Check sheet for the modelled part. Datum: model origin and axes. Units: mm. A direction names the side the tool comes from. Give positions to 0.01 mm unless a question says otherwise; leave off trailing zeros. Loops run counter-clockwise (first coordinate to the right, second up) from the corner with the lowest first, then second, coordinate; pieces in that order, holes last.
```python
from build123d import *

# Parameters (mm, degrees)
SKETCH_10_R         = 1.65
EXTRUDE_1_DEPTH     = 3
EXTRUDE_START       = 3
EXTRUDE_2_DEPTH     = 7
EXTRUDE_3_DEPTH     = 13
CHAMFER_1_SIZE      = 7
EXTRUDE_5_DEPTH     = 10
EXTRUDE_START_2     = -1.1
SKETCH_16_R         = 1.65
EXTRUDE_6_DEPTH     = 4.1
EXTRUDE_7_DEPTH     = 16
SKETCH_18_W         = 21
SKETCH_18_H         = 15.2
CUT_EXTRUDE_1_DEPTH = 14.1
FILLET_1_R          = 1


with BuildPart() as part:
    # 草图10 → 凸台-拉伸1 (new body)
    with BuildSketch(Plane.XY):
        Polygon((-78.55, -32.8), (-46.235028843, -32.8), (38.364971157, 51.8), (78.55, 51.8), (78.55, 32.8), (46.235028843, 32.8), (-38.364971157, -51.8), (-78.55, -51.8), align=None)
        with Locations((-68.55, -42.3)):
            Circle(SKETCH_10_R, mode=Mode.SUBTRACT)
        with Locations((68.55, 42.3)):
            Circle(SKETCH_10_R, mode=Mode.SUBTRACT)
    extrude(amount=EXTRUDE_1_DEPTH)

    # 草图11 → 凸台-拉伸2 (add)
    with BuildSketch(Plane.XY.offset(EXTRUDE_START)):
        Polygon((-59.55, -32.8), (-59.55, -51.8), (-38.364971157, -51.8), (46.235028843, 32.8), (57.55, 32.8), (57.55, 51.8), (38.364971157, 51.8), (-46.235028843, -32.8), align=None)
    extrude(amount=EXTRUDE_2_DEPTH)

    # 草图12 → 凸台-拉伸3 (add)
    with BuildSketch(Plane.XY.offset(EXTRUDE_START)):
        Polygon((-78.55, -32.8), (-46.235028843, -32.8), (38.364971157, 51.8), (78.55, 51.8), (78.55, 48.8), (39.607611845, 48.8), (-44.992388155, -35.8), (-78.55, -35.8), align=None)
        Polygon((-78.55, -48.8), (-78.55, -51.8), (-38.364971157, -51.8), (46.235028843, 32.8), (78.55, 32.8), (78.55, 35.8), (44.992388155, 35.8), (-39.607611845, -48.8), align=None)
    extrude(amount=EXTRUDE_3_DEPTH)

    # 倒角1
    chamfer_1_edges = [part.edges().sort_by_distance(p)[0] for p in [
        (57.55, 42.3, 10),
        (-59.55, -42.3, 10),
    ]]
    chamfer(chamfer_1_edges, length=CHAMFER_1_SIZE - 0.0001)  # a hair under: the kernel refuses the full size

    # 草图15 → 凸台-拉伸5 (add)
    with BuildSketch(Plane.XY.offset(3)):
        Polygon((-55.55, -35.8), (-55.55, -39.8), (-43.335533906, -39.8), (41.264466094, 44.8), (53.55, 44.8), (53.55, 48.8), (39.607611845, 48.8), (-44.992388155, -35.8), align=None)
        Polygon((-55.55, -44.8), (-55.55, -48.8), (-39.607611845, -48.8), (44.992388155, 35.8), (53.55, 35.8), (53.55, 39.8), (43.335533906, 39.8), (-41.264466094, -44.8), align=None)
    extrude(amount=EXTRUDE_5_DEPTH)

    # 草图16 → 凸台-拉伸6 (add)
    with BuildSketch(Plane.XY.offset(EXTRUDE_START_2)):
        Polygon((-78.55, -32.8), (-78.55, -51.8), (-38.364971157, -51.8), (45.135028843, 31.7), (78.55, 31.7), (78.55, 52.9), (39.464971157, 52.9), (-46.235028843, -32.8), align=None)
        with Locations((-68.55, -42.3)):
            Circle(SKETCH_16_R, mode=Mode.SUBTRACT)
        with Locations((68.55, 42.3)):
            Circle(SKETCH_16_R, mode=Mode.SUBTRACT)
    extrude(amount=EXTRUDE_6_DEPTH)

    # 草图17 → 凸台-拉伸7 (add)
    with BuildSketch(Plane.XY):
        Polygon((78.55, 52.9), (78.55, 48.8), (39.607611845, 48.8), (37.486291501, 50.921320344), (39.464971157, 52.9), align=None)
        Polygon((78.55, 31.7), (45.135028843, 31.7), (43.013708499, 33.821320344), (44.992388155, 35.8), (78.55, 35.8), align=None)
    extrude(amount=EXTRUDE_7_DEPTH)

    # 草图18 → 切除-拉伸1 (cut)
    with BuildSketch(Plane.XY.offset(16)):
        with Locations((68.05, 42.3)):
            Rectangle(SKETCH_18_W, SKETCH_18_H)
    extrude(amount=-CUT_EXTRUDE_1_DEPTH, mode=Mode.SUBTRACT)


with BuildPart() as cut_extrude_1_kept_piece:
    # of the separate pieces the step leaves, the one the design keeps (cut_extrude_1_pieces_kept)
    add(part.part.solids().sort_by_distance((-59.55, -48.8, 3.0001))[0])

    # 圆角1
    fillet_1_edges = [cut_extrude_1_kept_piece.edges().sort_by_distance(p)[0] for p in [
        (-46.235028843, -32.8, 7.45),
        (-38.364971157, -51.8, 7.45),
        (-43.335533906, -39.8, 11.5),
        (41.264466094, 44.8, 11.5),
        (-41.264466094, -44.8, 11.5),
        (43.335533906, 39.8, 11.5),
        (45.135028843, 31.7, 7.45),
        (39.464971157, 52.9, 7.45),
        (39.607611845, 48.8, 14.5),
        (-44.992388155, -35.8, 14.5),
        (-39.607611845, -48.8, 14.5),
        (44.992388155, 35.8, 14.5),
    ]]
    fillet(fillet_1_edges, radius=FILLET_1_R)


solid = cut_extrude_1_kept_piece.part
```
(1) Section check D-D on z = 4.75. Record the boundary of the cut face in (x, y).
(2) Material ranges on line 1 (Y direction, x = -68.55, z = 0.7); line 2 (Y direction, x = 68.55, z = 0.05); line 3 (X direction, y = 35, z = 15), recorded low to high.
(3) Section check A-A on x = 68.55. Record the boundary of the cut face in (y, z).
(4) Section check C-C on y = 42.3. Record the boundary of the cut face in (x, z), plus the area to 3 significant figures.
(5) Release check for a two-part mould opening along Y. For faces 1 (the face through (-65, -35.8, 9)), 2 (the face through (78.55, 42.2, 1.6)), 3 (the face through (-62, -32.8, 7)), 4 (the face through (67.9, 44.1, 1.9)) record: pulls with the +Y half, pulls with the -Y half, needs draft (parallel to the pull), parting line crosses it, or undercut.
(6) Gauge pin test, flat ends, axial feed: pin 1 Ø10 at (x, z) = (29, 3.5) entering from +Y (3 decimals); pin 2 Ø4.5 at (y, z) = (-46, 9) entering from -X; pin 3 Ø3 at (x, z) = (-48.5, 10.5) entering from +Y. Record the tip position at first contact, or that the pin passes through.
(7) Section check B-B on x = -68.55. Record the boundary of the cut face in (y, z).
(8) Access from +Z, -Z, +X, -X, +Y, -Y to the whole of each face (thin tool, end or side, straight path). Record for faces 5 (the face through (53.55, 38, 10)), 6 (the face through (-55.55, -38, 10)), 7 (the face through (-1, 5, 13)).
Computed values:
1. outline: (-78.55, -51.8) - (-38.78, -51.8) arc R1 ccw to (-38.07, -51.51) - (44.84, 31.41) arc R1 cw to (45.55, 31.7) - (78.55, 31.7) - (78.55, 34.7) - (57.55, 34.7) - (57.55, 35.8) - (55.8, 35.8) - (55.8, 48.8) - (57.55, 48.8) - (57.55, 49.9) - (78.55, 49.9) - (78.55, 52.9) - (39.88, 52.9) arc R1 ccw to (39.17, 52.61) - (-45.94, -32.51) arc R1 cw to (-46.65, -32.8) - (-78.55, -32.8) - (-78.55, -35.8) - (-57.8, -35.8) - (-57.8, -48.8) - (-78.55, -48.8) - close
2. line 1: y = -51.8 to -43.95, -40.65 to -32.8
2. line 2: y = 31.7 to 40.65, 43.95 to 52.9
2. line 3: x = 21.56 to 25.81, 44.19 to 57.55
3. outline: (31.7, -1.1) - (40.65, -1.1) - (40.65, 1.9) - (34.7, 1.9) - (34.7, 16) - (31.7, 16) - close; (43.95, -1.1) - (52.9, -1.1) - (52.9, 16) - (49.9, 16) - (49.9, 1.9) - (43.95, 1.9) - close
4. outline: (28.86, -1.1) - (66.9, -1.1) - (66.9, 1.9) - (57.55, 1.9) - (57.55, 3) - (50.55, 10) - (38.76, 10) - (38.76, 13) - (33.11, 13) - (33.11, 16) - (28.86, 16) - close; (70.2, -1.1) - (78.55, -1.1) - (78.55, 1.9) - (70.2, 1.9) - close
4. area: 389 mm2
5. face 1: undercut
5. face 2: needs draft
5. face 3: pulls with the +Y half
5. face 4: undercut
6. pin 1: stops at y = 47.435
6. pin 2: stops at x = -55.8
6. pin 3: stops at y = -32.8
7. outline: (-51.8, -1.1) - (-43.95, -1.1) - (-43.95, 3) - (-48.8, 3) - (-48.8, 16) - (-51.8, 16) - close; (-40.65, -1.1) - (-32.8, -1.1) - (-32.8, 16) - (-35.8, 16) - (-35.8, 3) - (-40.65, 3) - close
8. face 5: +Z, +X
8. face 6: +Z, -X
8. face 7: +Z
